Part print with two shaded views. Sizes in mm from the minimum x, y, z corner. A direction names the side the tool comes from. Round coordinates to 2 decimals unless told otherwise and drop trailing zeros. Write each loop counter-clockwise with the first axis right and the second up, starting at its lowest first coordinate (ties: lowest second). Pieces come first, ordered by that corner, then holes. Notation, with made-up numbers: (-40, -14.75) - (-2, -14.75) arc R12 ccw to (-2, -9.75) - close; hole circle Ø6 at (13, -17.75). An arc over 180 degrees is marked (long way). Answer as a JSON object with one key per item and string values. Group by question number.
Item 1: Slice it at B-B, the plane x = 10.5. List the corners of the cut face in (y, z), then the cut area to 3 significant figures.
Item 2: Slice it at C-C, the plane y = 7. List the corners of the cut face in (x, z), then the cut area to 3 significant figures.
Item 3: Two-plate mould, pull along X, no slides. Class the marked faces 1, 2 and 3: +X half, -X half, draft (parallel to the pull), parting line (faces both ways), or undercut.
Item 4: Flat gauge pins, fed straight in: pin 1 (0.9 mm diameter, centred on y = 2, z = 1.5, fed in from +X); pin 2 (0.7 mm diameter, centred on x = 40, z = 1, fed in from -Y); pin 3 (1.5 mm diameter, centred on y = 18, z = 1.5, fed in from +X). Where does each tip first touch, or does it go through?
Item 5: Probe line 1 (X direction, y = 4.5, z = 0.5); line 2 (Y direction, x = 6.5, z = 1.1); line 3 (Y direction, x = 3, z = 0.85). List the from-to ranges inside material, lowest first. Write a range as from..to.
Item 6: Which spindle directions (+Z, -Z, +X, -X, +Y, -Y) get a long thin tool onto all of the face, cutting with end or side? Do the marked faces 4, 5 and 6. Say none if no direction does.
Item 7: Slice it at A-A, the plane z = 0.45. List the corners of the cut face in (x, y), then the cut area to 3 significant figures.
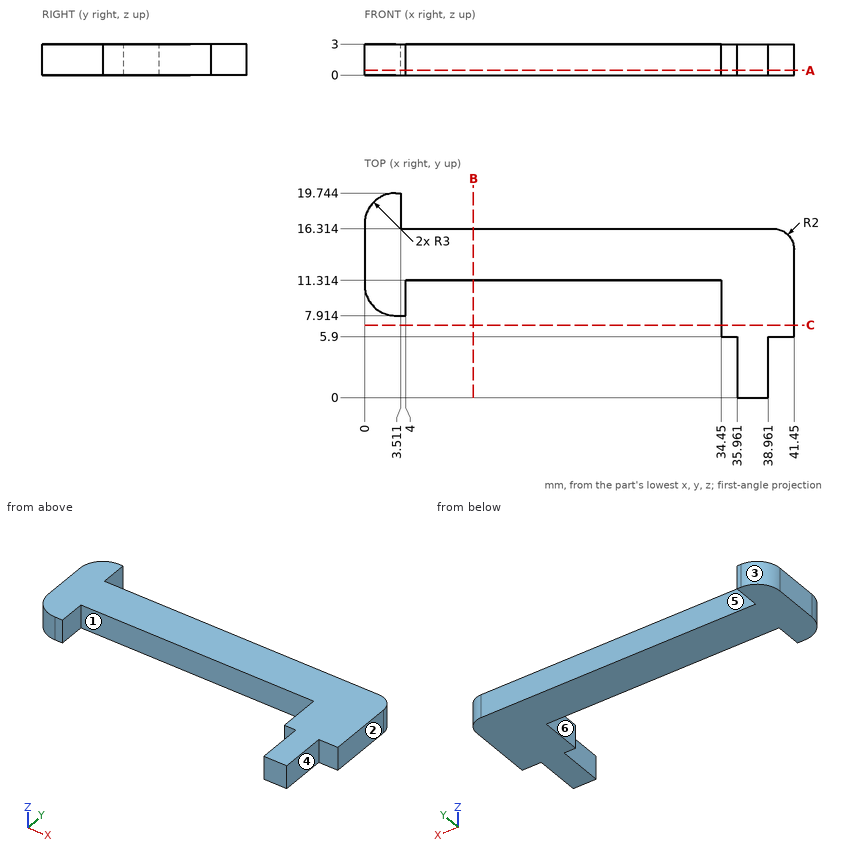
Geometry says:
{
 "1": {"outline": "(11.31, 0) - (16.31, 0) - (16.31, 3) - (11.31, 3) - close", "area": "15.0 mm^2"},
 "2": {"outline": "(34.45, 0) - (41.45, 0) - (41.45, 3) - (34.45, 3) - close", "area": "21.0 mm^2"},
 "3": {"face 1": "undercut", "face 2": "+X half", "face 3": "-X half"},
 "4": {"pin 1": "stops at x = 38.96", "pin 2": "stops at y = 5.9", "pin 3": "stops at x = 3.51"},
 "5": {"line 1": "x = 35.96..38.96", "line 2": "y = 11.31..16.31", "line 3": "y = 7.91..19.74"},
 "6": {"face 4": "+Z, -Z, +X, -Y", "face 5": "+Z, -Z, +X, +Y", "face 6": "+Z, -Z, -Y"},
 "7": {"outline": "(0, 10.91) arc R3 ccw to (3, 7.91) - (4, 7.91) - (4, 11.31) - (34.45, 11.31) - (34.45, 5.9) - (35.96, 5.9) - (35.96, 0) - (38.96, 0) - (38.96, 5.9) - (41.45, 5.9) - (41.45, 14.31) arc R2 ccw to (39.45, 16.31) - (3.51, 16.31) - (3.51, 19.74) - (3, 19.74) arc R3 ccw to (0, 16.74) - close", "area": "284 mm^2"}
}
